The listing builds one solid part. Answer for the finished solid, in the listing's coordinates (mm). Round coordinates to 2 decimals unless told otherwise and drop trailing zeros. Loops run counter-clockwise (first coordinate to the right, second up) from the corner with the lowest first, then second, coordinate; pieces in that order, holes last. Notation, with made-up numbers: (-5.75, 5) -> (45.25, 5) arc R16 cw to (45.25, 29) -> close; hole circle Ø3 at (73, 20.25). An arc over 180 degrees is marked (long way). Use a Markdown table: item, result. Add a question column.
Q1. Given pin 1 Ø1 at (x, y) = (22, -6.5) entering from -Z; pin 2 Ø6 at (x, y) = (46.5, -8.5) entering from -Z; pin 3 Ø6 at (y, z) = (-6.5, -253.5) entering from -X, each flat-ended and moving along its own axis, determine where each tip first touches the part or whether it passes through.
Q2. Section B-B on z = -293.5 is taken. Give the vertices of the cut face in (x, y), then the cut area to 3 significant figures.
Q3. Section A-A on x = 50 is taken. Give the vertices of the cut face in (y, z), then the cut area to 3 significant figures.
Q4. Section D-D on z = -276.5 is taken. Give the vertices of the cut face in (x, y), then the cut area to 3 significant figures.
Q5. Consider line 1 (Z direction, x = 53, y = -1.25); line 2 (Z direction, x = 65.5, y = -6.75); line 3 (X direction, y = -3.5, z = -305.5). Determine where each line is inside the solid, lowest interval first.
Q6. Section C-C on y = -6.75 is taken. Give the vertices of the cut face in (x, z), then the cut area to 3 significant figures.
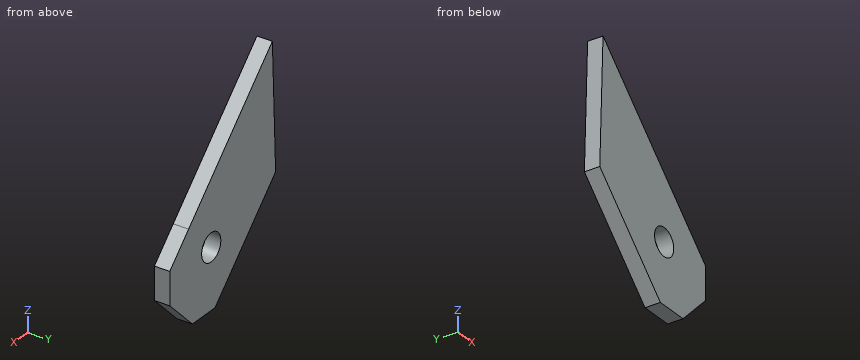
from build123d import *

# Parameters (mm, degrees)
F0_R     = 9
F1_DEPTH = 10
F2_SIZE  = 15


with BuildPart() as f1:
    # F0 (on Front) → F1 (new body)
    with BuildSketch(Plane.XZ):
        Polygon((106.8500287361, -307.0710678119), (78.5657574887, -278.7867965644), (0, -200.2210390757), (-3.0413549592, -282.0324978589), (64.4236218649, -349.4974746831), align=None)
        with Locations((57.3525540531, -300)):
            Circle(F0_R, mode=Mode.SUBTRACT)
    extrude(amount=F1_DEPTH)

    # F2
    f2_edges = [f1.edges().sort_by_distance(p)[0] for p in [
        (106.850029, -5, -307.071068),
        (64.423622, -5, -349.497475),
    ]]
    chamfer(f2_edges, length=F2_SIZE)


solid = f1.part
Checked values:
| question | item | result |
|---|---|---|
| 1 | pin 1 | stops at z = -307.57 |
| 1 | pin 2 | stops at z = -334.57 |
| 1 | pin 3 | stops at x = -2.09 |
| 2 | outline | (8.43, -10) -> (51.13, -10) -> (51.13, 0) -> (8.43, 0) -> close; (63.58, -10) -> (93.28, -10) -> (93.28, 0) -> (63.58, 0) -> close |
| 2 | area | 724 mm2 |
| 3 | outline | (-10, -335.07) -> (0, -335.07) -> (0, -305.19) -> (-10, -305.19) -> close; (-10, -294.81) -> (0, -294.81) -> (0, -250.22) -> (-10, -250.22) -> close |
| 3 | area | 745 mm2 |
| 4 | outline | (-2.84, -10) -> (76.28, -10) -> (76.28, 0) -> (-2.84, 0) -> close |
| 4 | area | 791 mm2 |
| 5 | line 1 | z = -338.07 to -307.88, -292.12 to -253.22 |
| 5 | line 2 | z = -338.89 to -303.82, -296.18 to -265.72 |
| 5 | line 3 | x = 20.43 to 50.23, 64.48 to 96.24 |
| 6 | outline | (-3.04, -282.03) -> (53.82, -338.89) -> (75.03, -338.89) -> (96.24, -317.68) -> (96.24, -296.46) -> (0, -200.22) -> close; hole circle Ø18 at (57.35, -300) |
| 6 | area | 6,920 mm2 |
